```python
from build123d import *

# Parameters (mm, degrees)
BOSS_EXTRUDE1_DEPTH = 4
SKETCH4_W           = 26
SKETCH4_H           = 14
BOSS_EXTRUDE2_DEPTH = 3
FILLET1_R           = 1
FILLET3_R           = 3
FILLET4_R           = 3
BOSS_EXTRUDE9_DEPTH = 14
FILLET5_R           = 2
FILLET6_R           = 2


# Some blends are built 0.0001 mm under size
with BuildPart() as part:
    # Sketch1 → Boss-Extrude1 (new body)
    with BuildSketch(Plane(origin=(0, 0, 0), x_dir=(-1, 0, 0), z_dir=(0, 0, -1))):
        with BuildLine():
            Line((27.500000074, -16.263075607), (27.500000074, 0))
            Line((27.500000074, 0), (-20.499999926, 0))
            Line((-20.499999926, 0), (-20.499999926, -15.701236215))
            ThreePointArc((-20.499999926, -15.701236215), (3.511255672, -15.020548898), (27.500000074, -16.263075607))
        make_face()
    extrude(amount=-BOSS_EXTRUDE1_DEPTH)

    # Sketch4 → Boss-Extrude2 (add)
    with BuildSketch(Plane.XY.offset(4)):
        with Locations((-3.500000074, -7)):
            Rectangle(SKETCH4_W, SKETCH4_H)
    extrude(amount=BOSS_EXTRUDE2_DEPTH)

    # Fillet1
    fillet1_edges = [part.edges().sort_by_distance(p)[0] for p in [
        (20.499999926, 0, 2),
        (-27.500000074, 0, 2),
        (20.499999926, -15.701236215, 2),
        (-27.500000074, -16.263075607, 2),
    ]]
    fillet(fillet1_edges, radius=FILLET1_R)

    # Fillet3
    fillet3_edges = [part.edges().sort_by_distance(p)[0] for p in [
        (-3.500000074, -14, 7),
        (-16.500000074, -7, 7),
        (9.499999926, -7, 7),
    ]]
    fillet(fillet3_edges, radius=FILLET3_R - 0.0001)  # a hair under: the kernel refuses the full size

    # Fillet4
    # the kernel refuses this fillet: 3 mm, written as the material it takes off along each edge
    with BuildSketch(Plane(origin=(-13.500000074, -11, 7), x_dir=(-1, 0, 0), z_dir=(0, 1, 0))) as fillet4_piece_1:
        with BuildLine():
            CenterArc((0.0001, -2.9999), 2.9999, 0, 90)
            Line((3, -2.9999), (3, 0))
            Line((3, 0), (0.0001, 0))
        make_face()
    revolve(axis=Axis((-13.500000074, -11, 7), (0, 0, 1)), revolution_arc=90, mode=Mode.SUBTRACT)
    with BuildSketch(Plane(origin=(6.499999926, -11, 7), x_dir=(0, -1, 0), z_dir=(-1, 0, 0))) as fillet4_piece_2:
        with BuildLine():
            CenterArc((0.0001, -2.9999), 2.9999, 0, 90)
            Line((3, -2.9999), (3, 0))
            Line((3, 0), (0.0001, 0))
        make_face()
    revolve(axis=Axis((6.499999926, -11, 7), (0, 0, 1)), revolution_arc=90, mode=Mode.SUBTRACT)
    with BuildSketch(Plane(origin=(9.499999926, -14, 4), x_dir=(0, 1, 0), z_dir=(0, 0, 1))) as fillet4_piece_3:
        with BuildLine():
            CenterArc((FILLET4_R, FILLET4_R), FILLET4_R, 180, 90)
            Line((0, FILLET4_R), (0, 0))
            Line((0, 0), (FILLET4_R, 0))
        make_face()
    extrude(amount=3, mode=Mode.SUBTRACT)
    with BuildSketch(Plane(origin=(-16.500000074, -14, 4), x_dir=(0, 1, 0), z_dir=(0, 0, 1))) as fillet4_piece_4:
        with BuildLine():
            CenterArc((FILLET4_R, -FILLET4_R), FILLET4_R, 90, 90)
            Line((0, -FILLET4_R), (0, 0))
            Line((0, 0), (FILLET4_R, 0))
        make_face()
    extrude(amount=3, mode=Mode.SUBTRACT)

    # Sketch21 → Boss-Extrude9 (add)
    with BuildSketch(Plane(origin=(0, 0, 0), x_dir=(1, 0, 0), z_dir=(0, 1, 0))):
        with BuildLine():
            Line((6.499999926, -7), (-13.500000074, -7))
            ThreePointArc((-13.500000074, -7), (-15.621320417, -6.121320344), (-16.500000074, -4))
            Line((-16.500000074, -4), (-16.500000074, -3))
            Line((-16.500000074, -3), (9.499999926, -3))
            Line((9.499999926, -3), (9.499999926, -4))
            ThreePointArc((9.499999926, -4), (8.62132027, -6.121320344), (6.499999926, -7))
        make_face()
    extrude(amount=BOSS_EXTRUDE9_DEPTH)

    # Fillet5
    fillet5_edges = [part.edges().sort_by_distance(p)[0] for p in [
        (-16.500000074, 14, 3.5),
        (-15.621320417, 14, 6.121320344),
        (9.499999926, 14, 3.5),
        (8.62132027, 14, 6.121320344),
        (-3.500000074, 14, 7),
    ]]
    fillet(fillet5_edges, radius=FILLET5_R)

    # Fillet6
    fillet6_edges = [part.edges().sort_by_distance(p)[0] for p in [
        (-3.500000074, 0, 3),
    ]]
    fillet(fillet6_edges, radius=FILLET6_R)


solid = part.part
```
Source: CAD feature listing. Evaluate the final solid. Frame: model axes, mm. A direction names the side the tool comes from. Round coordinates to 2 decimals unless told otherwise and drop trailing zeros. Write each loop counter-clockwise with the first axis right and the second up, starting at its lowest first coordinate (ties: lowest second). Pieces come first, ordered by that corner, then holes. Notation, with made-up numbers: M -9.75,57 L 36.25,57 A19 cw 36.25,77 Z; hole C 23,-37 d2. An arc over 180 degrees is marked long. Use CSV: the item, a comma, the result in double quotes. Start each with the question number.
Q1. First-contact query: P1, Ø4, axis at x = 0, z = 1, coming from the -Y side; P2, Ø1.5, axis at x = 7.5, y = -11.5, coming from the +Z side; P3, Ø6, axis at x = -9.5, y = 10, coming from the -Z side. Flat tips, straight axial feed; report the tip coordinate or a pass-through.
Q2. Cut plane C-C on z = 1.75. Output: boundary loops of the cut face in (x, y).
Q3. Access query for faces 1 (the face through (-3.8, 0, 0.6)), 2 (the face through (9.5, 5.5, 3.5)), 3 (the face through (-15.64, -5.42, 6.1)). Directions: +Z, -Z, +X, -X, +Y, -Y. A direction counts if a zero-diameter tool reaches every point of the face in a straight line with its end or side. Return the directions, or none.
Q4. Line query: line 1 (Z direction, x = -18.5, y = -15); line 2 (Z direction, x = -3, y = 9.5); line 3 (X direction, y = 3, z = 4). Output: solid intervals per line, ascending. Write a range as from..to.
Q5. Cut plane D-D on y = 10.5. Output: boundary loops of the cut face in (x, z), plus the area to 3 significant figures.
Results found:
1,P1,"y = -15.01"
1,P2,"z = 6.98"
1,P3,"z = 3"
2,outline,"M -27.5,-15.17 A1 ccw -26.41,-16.16 A300 cw 19.44,-15.63 A1 ccw 20.5,-14.63 L 20.5,-1 A1 ccw 19.5,0 L 9.5,0 L 9.5,0.15 L -16.5,0.15 L -16.5,0 L -26.5,0 A1 ccw -27.5,-1 Z"
3,face 1,"-Z, +Y"
3,face 2,"+Z, -Z, +X, +Y"
3,face 3,"+Z, -X, +Y, -Y"
4,line 1,"0..4"
4,line 2,"3..7"
4,line 3,"-16.5..9.5"
5,outline,"M -16.5,3 L 9.5,3 L 9.5,4 A3 ccw 6.5,7 L -13.5,7 A3 ccw -16.5,4 Z"
5,area,"100 mm^2"
